from build123d import *

# Parameters (mm, degrees)
F2_DEPTH = 4
F3_W     = 50
F3_H     = 14
F4_DEPTH = 2.1
F5_R     = 5


with BuildPart() as f2:
    # F1 (on Front) → F2 (new body)
    with BuildSketch(Plane.XZ):
        Polygon((-20, 0), (20, 0), (20, 74), (6, 74), (6, 76), (-6, 76), (-6, 74), (-20, 74), align=None)
    extrude(amount=F2_DEPTH)

    # F3 (on Top) → F4 (join)
    with BuildSketch(Plane.XY):
        with Locations((0, -2)):
            Rectangle(F3_W, F3_H)
    extrude(amount=F4_DEPTH)

    # F5
    f5_edges = [f2.edges().sort_by_distance(p)[0] for p in [
        (-25, -9, 1.05),
        (25, -9, 1.05),
        (25, 5, 1.05),
        (-25, 5, 1.05),
    ]]
    fillet(f5_edges, radius=F5_R)


solid = f2.part
Source: CAD feature listing. Evaluate the final solid. Frame: model axes, mm. A direction names the side the tool comes from. Coordinates: 2 decimals unless noted, no trailing zeros. Write each loop counter-clockwise with the first axis right and the second up, starting at its lowest first coordinate (ties: lowest second). Pieces come first, ordered by that corner, then holes. Notation, with made-up numbers: M 82.5,-31.75 L 135.5,-31.75 A26 cw 135.5,0.25 Z; hole C 78,86.25 d10. An arc over 180 degrees is marked long. Use a Markdown table: item, result.
1) Reachability of faces 1 (the flat face through (0, -4, 40)), 2 (the flat face through (0, 0, 40)), 3 (the flat face through (6, -2, 75)), 4 (the flat face through (-6, -2, 75)), 5 (the cylindrical face through (-24, 3, 1)) from +Z, -Z, +X, -X, +Y, -Y: full face, straight path, thin tool, end or side. Return the list, or none.
Conclusion:
| item | result |
|---|---|
| face 1 | +Z, +X, -X, -Y |
| face 2 | +Z, +X, -X, +Y |
| face 3 | +Z, +X, +Y, -Y |
| face 4 | +Z, -X, +Y, -Y |
| face 5 | +Z, -Z, -X, +Y |
2) Ray query, L1, parallel to X at y = -2.25, z = 28; L2, parallel to Z at x = -20, y = 3; L3, parallel to Y at x = -16.5, z = 69.5. Return the intervals inside material, ascending.
Conclusion:
| item | result |
|---|---|
| L1 | x = -20 to 20 |
| L2 | z = 0 to 2.1 |
| L3 | y = -4 to 0 |
3) First-contact query: pin 1 Ø8 at (y, z) = (-1.5, 25.5) entering from +X; pin 2 Ø6 at (y, z) = (-1.5, 30) entering from -X; pin 3 Ø3 at (x, y) = (10, -2) entering from +Z. Flat tips, straight axial feed; report the tip coordinate or a pass-through.
Conclusion:
| item | result |
|---|---|
| pin 1 | stops at x = 20 |
| pin 2 | stops at x = -20 |
| pin 3 | stops at z = 74 |
4) Section C-C, the plane z = 23.5. Output: boundary loops of the cut face in (x, y), then the cut area to 3 significant figures.
Conclusion:
| item | result |
|---|---|
| outline | M -20,-4 L 20,-4 L 20,0 L -20,0 Z |
| area | 160 mm^2 |
5) Section A-A, the plane x = 12. Output: boundary loops of the cut face in (y, z).
Conclusion:
| item | result |
|---|---|
| outline | M -9,0 L 5,0 L 5,2.1 L 0,2.1 L 0,74 L -4,74 L -4,2.1 L -9,2.1 Z |
6) Section D-D, the plane x = 4. Output: boundary loops of the cut face in (y, z), then the cut area to 3 significant figures.
Conclusion:
| item | result |
|---|---|
| outline | M -9,0 L 5,0 L 5,2.1 L 0,2.1 L 0,76 L -4,76 L -4,2.1 L -9,2.1 Z |
| area | 325 mm^2 |
7) Section B-B, the plane y = -2.75. Output: boundary loops of the cut face in (x, z).
Conclusion:
| item | result |
|---|---|
| outline | M -25,0 L 25,0 L 25,2.1 L 20,2.1 L 20,74 L 6,74 L 6,76 L -6,76 L -6,74 L -20,74 L -20,2.1 L -25,2.1 Z |
